CAD build for the part. Positions are in the model's coordinates, mm. Face numbers are marked on the shaded views. Coordinates: 2 decimals unless noted, no trailing zeros. Loops run counter-clockwise (first coordinate to the right, second up) from the corner with the lowest first, then second, coordinate; pieces in that order, holes last. Notation, with made-up numbers: (6.25, 20.5) -> (12.25, 20.5) arc R9 ccw to (12.25, 28.5) -> close; hole circle Ø9 at (53, -10). An arc over 180 degrees is marked (long way). Write each question's results on one line, items separated by ' | '.
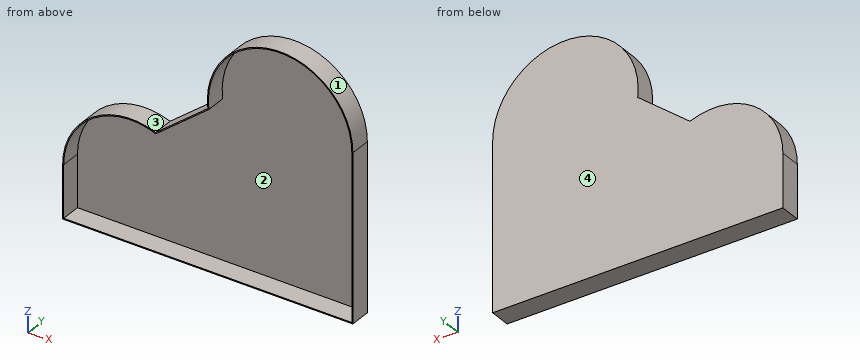
from build123d import *

# Parameters (mm, degrees)
F1_DEPTH = 50
F2_T     = -2.5


with BuildPart() as f1:
    # F0 (on Front) → F1 (new body)
    with BuildSketch(Plane.XZ):
        with BuildLine():
            ThreePointArc((155.2564352751, 163.4969860315), (5.8915510694, 146.0091765296), (-64.1858130693, 12.949584052))
            Line((-64.1858130693, 12.949584052), (-64.1858130693, -112.6743033528))
            Line((-64.1858130693, -112.6743033528), (621.2269067764, -112.6743033528))
            Line((621.2269067764, -112.6743033528), (621.2269067764, 280.9008359909))
            ThreePointArc((621.2269067764, 280.9008359909), (439.8735747108, 452.4664689198), (278.6230742931, 261.8829607964))
            Line((278.6230742931, 261.8829607964), (155.2564352751, 163.4969860315))
        make_face()
    extrude(amount=F1_DEPTH)

    # F2
    f2_openings = [f1.faces().sort_by_distance(p)[0] for p in [
        (335.096712, -50, 111.093297),
    ]]
    offset(amount=F2_T, openings=f2_openings, kind=Kind.INTERSECTION)


solid = f1.part
1) Two-plate mould, pull along X, no slides. Class the marked faces 1, 2, 3 and 4: pulls with the +X half, pulls with the -X half, needs draft (parallel to the pull), parting line crosses it, or undercut.
Outcome:
face 1: parting line crosses it | face 2: undercut | face 3: undercut | face 4: needs draft
2) Slice it at B-B (z = -4). Write the cut outline in (x, y).
Outcome:
outline: (-64.19, -50) -> (-61.69, -50) -> (-61.69, -2.5) -> (618.73, -2.5) -> (618.73, -50) -> (621.23, -50) -> (621.23, 0) -> (-64.19, 0) -> close
3) Pin check, flat tips, straight feed: pin 1 (1 mm diameter, centred on x = 182, y = -39.5, fed in from +Z); pin 2 (3 mm diameter, centred on y = -10.5, z = 227, fed in from -X); pin 3 (14 mm diameter, centred on x = 403.5, y = -37.5, fed in from +Z). Stop position of each tip, or through.
Outcome:
pin 1: stops at z = 185.22 | pin 2: stops at x = 233 | pin 3: stops at z = 448.27
4) Drill centre lines: L1, parallel to X at y = -23, z = 277; L2, parallel to X at y = -22, z = -68; L3, parallel to Y at x = 179, z = 61. Where is each one in solid material? Low to high. Write a range as from..to.
Outcome:
L1: x = 277.61..280.11, 618.73..621.23 | L2: x = -64.19..-61.69, 618.73..621.23 | L3: y = -2.5..0
5) Slice it at C-C (x = 531.5). Write the cut outline in (y, z), then the cut area to 3 significant figures.
Outcome:
outline: (-50, -112.67) -> (0, -112.67) -> (0, 431.85) -> (-50, 431.85) -> (-50, 428.99) -> (-2.5, 428.99) -> (-2.5, -110.17) -> (-50, -110.17) -> close | area: 1,620 mm^2
6) Slice it at A-A (y = -35). Write the cut outline in (x, z), then the cut area to 3 significant figures.
Outcome:
outline: (-64.19, -112.67) -> (621.23, -112.67) -> (621.23, 280.9) arc R171.83 ccw (long way) to (278.62, 261.88) -> (155.26, 163.5) arc R161.36 ccw to (-64.19, 12.95) -> close; hole (-61.69, -110.17) -> (618.73, -110.17) -> (618.73, 280.9) arc R169.33 ccw (long way) to (281.27, 260.79) -> (155.69, 160.64) arc R158.86 ccw to (-61.69, 12.95) -> close | area: 5,560 mm^2
